from build123d import *

# Parameters (mm, degrees)
F1_DEPTH = 320
F2_W     = 308
F2_H     = 30
F3_DEPTH = 306
F4_R     = 4


with BuildPart() as f1:
    # F0 (on Right) → F1 (new body)
    with BuildSketch(Plane.YZ):
        Polygon((0, -312), (0, 0), (-430, 0), (-400, -312), align=None)
    extrude(amount=F1_DEPTH)

    # F2 (on face) → F3 (cut, through all)
    with BuildSketch(Plane(origin=(0, 0, -312), x_dir=(1, 0, 0), z_dir=(0, 0, -1))):
        with Locations((160, 415)):
            Rectangle(F2_W, F2_H)
    extrude(amount=-F3_DEPTH, mode=Mode.SUBTRACT)

    # F4
    f4_edges = [f1.edges().sort_by_distance(p)[0] for p in [
        (0, -215, 0),
        (320, -215, 0),
    ]]
    fillet(f4_edges, radius=F4_R)


solid = f1.part
Can you work these out from the model? Positions are in its coordinate system, mm. A direction names the side the tool comes from. Coordinates: 2 decimals unless noted, no trailing zeros. Write each loop counter-clockwise with the first axis right and the second up, starting at its lowest first coordinate (ties: lowest second). Pieces come first, ordered by that corner, then holes. Notation, with made-up numbers: (32.25, 50.5) -> (47.25, 50.5) arc R21 ccw to (47.25, 72.5) -> close; hole circle Ø9 at (-33, -33). An arc over 180 degrees is marked (long way). Write each question's results on one line, items separated by ' | '. Start each with the question number.
Item 1: If we section it at A-A, the plane x = 115: Write out the boundary of the cut face in (y, z), and give its area (3 significant figures).
Item 2: If we section it at B-B, the plane z = -162.5: Write out the boundary of the cut face in (x, y) (3 decimals), and give its area (3 significant figures).
Item 3: I'm going to push flat-ended pins straight in: P1, Ø14.5, axis at x = 178.5, y = -421, coming from the -Z side; P2, Ø10, axis at x = 180.5, z = -131.5, coming from the -Y side; P3, Ø9, axis at y = -415.5, z = -217, coming from the -X side (1 decimal). Where does each tip first touch, or does it pass through?
Item 4: On a 3-axis mill with a long thin cutter (end or side, diameter ignored), from which of +Z, -Z, +X, -X, +Y, -Y can I reach the whole of each face in a straight line? I mean faces 1 (the flat face through (314, -408, -93)), 2 (the flat face through (0, -218, -156)). Say none if no direction works.
Item 5: Please list where this line runs through material, in increasing order: probe 1 along Y at (x, z) = (170, -23.5).
Item 6: If we section it at C-C, the plane z = -104.5: Write out the boundary of the cut face in (x, y).
Answer block:
1) outline: (-430, 0) -> (-429.42, -6) -> (-400, -6) -> (-400, -312) -> (0, -312) -> (0, 0) -> close | area: 125,000 mm²
2) outline: (0, -414.375) -> (6, -414.375) -> (6, -400) -> (314, -400) -> (314, -414.375) -> (320, -414.375) -> (320, 0) -> (0, 0) -> close | area: 128,000 mm²
3) P1: z = -6 | P2: y = -400 | P3: through
4) face 1: -Z, -Y | face 2: +Z, -Z, -X, +Y, -Y
5) probe 1: -400 to 0
6) outline: (0, -419.95) -> (6, -419.95) -> (6, -400) -> (314, -400) -> (314, -419.95) -> (320, -419.95) -> (320, 0) -> (0, 0) -> close
